```python
from build123d import *

# Parameters (mm, degrees)
SKETCH1_W           = 34.63
SKETCH1_H           = 10
SKETCH1_R           = 1.85
BOSS_EXTRUDE1_DEPTH = 20
CHAMFER1_SIZE       = 1
SKETCH2_R           = 12
CUT_EXTRUDE1_DEPTH  = 27.9222812
BOSS_EXTRUDE2_DEPTH = 26
SKETCH5_R           = 2.25
CUT_EXTRUDE3_DEPTH  = 51.598783582
CHAMFER2_SIZE       = 1
CHAMFER3_SIZE       = 28
CHAMFER4_SIZE       = 22.238414528
CHAMFER4_SIZE_2     = 15


with BuildPart() as part:
    # Sketch1 → Boss-Extrude1 (new body)
    with BuildSketch(Plane.XY):
        Rectangle(SKETCH1_W, SKETCH1_H)
        with Locations((-11.315, 0)):
            Circle(SKETCH1_R, mode=Mode.SUBTRACT)
        with Locations((11.315, 0)):
            Circle(SKETCH1_R, mode=Mode.SUBTRACT)
    extrude(amount=BOSS_EXTRUDE1_DEPTH)

    # Chamfer1
    chamfer1_edges = [part.edges().sort_by_distance(p)[0] for p in [
        (-13.165, 0, 0),
        (9.465, 0, 0),
    ]]
    chamfer(chamfer1_edges, length=CHAMFER1_SIZE)

    # Sketch2 → Cut-Extrude1 (cut, through all)
    with BuildSketch(Plane.XY.offset(20)):
        with Locations((0, -14)):
            Circle(SKETCH2_R)
    extrude(amount=-CUT_EXTRUDE1_DEPTH, mode=Mode.SUBTRACT)

    # Sketch3 → Boss-Extrude2 (add)
    with BuildSketch(Plane(origin=(0, 5, 0), x_dir=(1, 0, 0), z_dir=(0, 1, 0))):
        Polygon((-17.315, 0), (-17.315, -20), (11.315, -20), (17.315, -20), (17.315, 0), align=None)
    extrude(amount=BOSS_EXTRUDE2_DEPTH)

    # Sketch5 → Cut-Extrude3 (cut, through all)
    with BuildSketch(Plane(origin=(17.315, 0, 0), x_dir=(0, 0, -1), z_dir=(1, 0, 0))):
        with Locations((-12, 20.5)):
            Circle(SKETCH5_R)
    extrude(amount=-CUT_EXTRUDE3_DEPTH, mode=Mode.SUBTRACT)

    # Chamfer2
    chamfer2_edges = [part.edges().sort_by_distance(p)[0] for p in [
        (17.315, 20.5, 14.25),
    ]]
    chamfer(chamfer2_edges, length=CHAMFER2_SIZE)

    # Chamfer3
    # the kernel refuses this chamfer: 28 mm, written as the material it takes off along each edge
    with BuildSketch(Plane(origin=(-17.315, 31, -72.007123663), x_dir=(0.9996219169112968, 0.027495876610586365, 0), z_dir=(0, 0, 1))) as chamfer3_piece_1:
        Polygon((CHAMFER3_SIZE * 0.999621916911, -CHAMFER3_SIZE * 0.0274958766106), (-CHAMFER3_SIZE * 0.0274958766106, -CHAMFER3_SIZE * 0.999621916911), (0, 0), align=None)
    extrude(amount=164.014247326, mode=Mode.SUBTRACT)

    # Chamfer4
    # the kernel refuses this chamfer: 22.238414528, 15 mm, written as the material it takes off along each edge
    with BuildSketch(Plane(origin=(-17.315, 60.453144221, 20), x_dir=(0.9997657259302418, 0, 0.021644705014774085), z_dir=(0, -1, 0))) as chamfer4_piece_1:
        Polygon((CHAMFER4_SIZE * 0.999765725916, -CHAMFER4_SIZE * 0.0216447050145), (-CHAMFER4_SIZE_2 * 0.0216447050148, -CHAMFER4_SIZE_2 * 0.99976572593), (0, 0), align=None)
    extrude(amount=122.906288442, mode=Mode.SUBTRACT)


solid = part.part
```
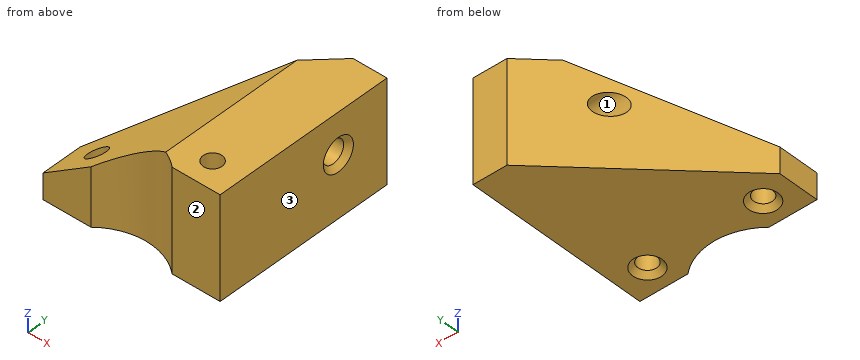
Model file for the job. Use its own axes, mm. Face numbers are marked on the shaded views. Coordinates: 2 decimals unless noted, no trailing zeros. Write each loop counter-clockwise with the first axis right and the second up, starting at its lowest first coordinate (ties: lowest second). Pieces come first, ordered by that corner, then holes. Notation, with made-up numbers: (68.5, -26) - (114.5, -26) arc R30 cw to (114.5, 4) - close; hole circle Ø5 at (75.25, 23.25). An arc over 180 degrees is marked (long way). One line per item, written item: value. Start each with the question number.
1. Probe line 1 (Z direction, x = 9.5, y = 20.5); line 2 (Y direction, x = 10.25, z = 12) (3 decimals); line 3 (Y direction, x = 3.5, z = 12) (3 decimals). List the from-to ranges inside material, lowest first. Write a range as from..to.
2. Slice it at B-B (y = 0). Write the cut outline in (x, z) (3 decimals).
3. Flat gauge pins, fed straight in: pin 1 (4 mm diameter, centred on y = 20.5, z = 12, fed in from -X); pin 2 (3 mm diameter, centred on y = 20, z = 8, fed in from -X) (3 decimals); pin 3 (5 mm diameter, centred on x = 11.315, y = 0, fed in from -Z); pin 4 (4 mm diameter, centred on y = 24.5, z = 2, fed in from -X) (3 decimals). Where does each tip first touch, or does it go through?
4. Slice it at D-D (z = 16.5). Write the cut outline in (x, y) (3 decimals), plus the area to 3 significant figures.
5. Slice it at A-A (z = 12). Write the cut outline in (x, y) (3 decimals).
6. Mould opens along Y. For the marked faces 1, 2 and 3 say: released by +Y, released by -Y, zero draft, split by the parting line, or undercut.
7. Slice it at C-C (y = 20.5). Write the cut outline in (x, z) (3 decimals).
Answers below:
1. line 1: z = 0..9.75, 14.25..20
1. line 2: y = -5..-1.513, 1.513..18.25, 22.75..30.565
1. line 3: y = -2.522..18.25, 22.75..23.815
2. outline: (-17.315, 0) - (-14.165, 0) - (-13.165, 1) - (-13.165, 7.799) - (-17.315, 5) - close; (-9.465, 1) - (-8.465, 0) - (8.465, 0) - (9.465, 1) - (9.465, 20) - (4.923, 20) - (-9.465, 10.295) - close; (13.165, 1) - (14.165, 0) - (17.315, 0) - (17.315, 20) - (13.165, 20) - close
3. pin 1: passes through
3. pin 2: stops at x = -1.815
3. pin 3: stops at z = 0.35
3. pin 4: stops at x = 2.185
4. outline: (-0.266, -2.003) arc R12 cw to (7.937, -5) - (17.315, -5) - (17.315, 31) - (10.685, 31) - (-0.266, 20.049) - close; hole circle Ø3.7 at (11.315, 0)
4. area: 545 mm^2
5. outline: (-6.937, -4.208) arc R12 cw to (7.937, -5) - (17.315, -5) - (17.315, 17.25) - (16.315, 18.25) - (-2.065, 18.25) - (-6.937, 13.378) - close; (2.435, 22.75) - (16.315, 22.75) - (17.315, 23.75) - (17.315, 31) - (10.685, 31) - close; hole circle Ø3.7 at (11.315, 0)
6. face 1: undercut
6. face 2: released by -Y
6. face 3: zero draft
7. outline: (0.185, 0) - (17.315, 0) - (17.315, 8.75) - (16.315, 9.75) - (0.185, 9.75) - close; (0.185, 14.25) - (16.315, 14.25) - (17.315, 15.25) - (17.315, 20) - (4.923, 20) - (0.185, 16.804) - close
